The model under review builds one solid part; all positions refer to its coordinate system, in mm. A direction names the side the tool comes from. Give positions to 0.01 mm unless a question says otherwise; leave off trailing zeros. Loops run counter-clockwise (first coordinate to the right, second up) from the corner with the lowest first, then second, coordinate; pieces in that order, holes last. Notation, with made-up numbers: M 65.25,-28 L 109.25,-28 A19 cw 109.25,-9 Z; hole C -11,36 d11. An arc over 180 degrees is marked long. Return JSON: item names as keys, results as strings.
Autodesk Inventor part; units mm, degrees
ref_plane "YZ Plane" through (0, 0, 0) normal (1, 0, 0) x (0, 1, 0)
ref_plane "XZ Plane" through (0, 0, 0) normal (0, 1, 0) x (-1, 0, 0)
ref_plane "XY Plane" through (0, 0, 0) normal (0, 0, 1) x (1, 0, 0)
sketch "Sketch1" plane through (0, 0, 0) normal (0, 0, 1) x (1, 0, 0)
  line L0 (0, 0) -> (2, 0)
  line L1 (2, 0) -> (2, 10)
  line L2 (2, 10) -> (28, 10)
  line L3 (28, 10) -> (28, 0)
  line L4 (28, 0) -> (30, 0)
  line L5 (30, 0) -> (30, 12)
  line L6 (30, 12) -> (0, 12)
  line L7 (0, 12) -> (0, 0)
  line L8 (30, 15) -> (0, 15)
  dimension "d0" = 2
  dimension "d1" = 10
  dimension "d2" = 26
  dimension "d3" = 2
  dimension "d4" = 12
  dimension "d5" = 3
  dimension "d6" = 30
revolve "Revolution1" add sketch "Sketch1" angle 360 about axis through (30, 15, 0) along (-1, 0, 0)
sketch "Sketch2" plane through (0, 15, 0) normal (-1, 0, 0) x (0, 0, 1)
  circle A0 centre (7, 0) radius 2
  circle A1 centre (-7, 0) radius 2
  circle A2 centre (0, 7) radius 2
  circle A3 centre (0, -7) radius 2
  point P0 (0, -15)
  point P1 (0, 0)
  dimension "d8" = 4
  dimension "d10" = 4
  dimension "d13" = 4
  dimension "d14" = 4
  dimension "d17" = 7
  dimension "d18" = 7
  dimension "d19" = 7
  dimension "d20" = 7
sketch "Sketch3" plane through (0, 15, 0) normal (-1, 0, 0) x (0, 0, 1)
  point P0 (0, -15)
extrude "Extrusion1" cut sketch "Sketch2" against normal blind 2
sketch "Sketch4" plane through (30, 15, 0) normal (1, 0, 0) x (0, 0, -1)
  circle A0 centre (13, 0) radius 1
  circle A1 centre (-6, 0) radius 1
  point P0 (0, -15)
  point P1 (0, 0)
  dimension "d23" = 2
  dimension "d24" = 2
  dimension "d25" = 6
  dimension "d26" = 13
extrude "Extrusion2" cut sketch "Sketch4" against normal blind 2
properties part number "Spool1"
1) Insertion check: pin 1 (10 mm diameter, centred on y = 8, z = 4.5, fed in from -X); pin 2 (6 mm diameter, centred on x = 11.5, y = 6.5, fed in from -Z); pin 3 (2 mm diameter, centred on y = 8.5, z = -0.5, fed in from -X); pin 4 (5 mm diameter, centred on x = 24.5, z = -4, fed in from +Y). Each pin has a flat end and moves straight along its axis. Give the tip position at first contact, or say it passes through.
From the geometry:
{"pin 1": "x = 0", "pin 2": "through", "pin 3": "x = 28", "pin 4": "y = 19.77"}
2) Tool access review of faces 5 (the face through (29, 14, -13)), 6 (the face through (2, 19, 4)), 7 (the face through (1, 10, 0)), 8 (the face through (15, 18, 0)): name each direction out of +Z, -Z, +X, -X, +Y, -Y from which nothing blocks a thin tool from reaching the whole face with its end or side.
From the geometry:
{"face 5": "+X", "face 6": "none", "face 7": "-X", "face 8": "+X, -X"}
3) The part is to be moulded in two halves that separate along Y. For faces 1 (the face through (1, 17, 7)), 2 (the face through (0.986, 20.226, 0.923)), 3 (the face through (1, 27, 9)), 4 (the face through (30, 15, 4)), say which applies: released by +Y, released by -Y, zero draft, split by the parting line, or undercut.
From the geometry:
{"face 1": "undercut", "face 2": "undercut", "face 3": "split by the parting line", "face 4": "zero draft"}
4) Consider section C-C on y = 8. Write out the cut boundary in (x, z), then the cut area to 3 significant figures.
From the geometry:
{"outline": "M 0,-13.27 L 2,-13.27 L 2,-2 L 0,-2 Z; M 0,2 L 2,2 L 2,13.27 L 0,13.27 Z; M 28,-13.27 L 30,-13.27 L 30,13.27 L 28,13.27 Z", "area": "98.1 mm²"}
5) Consider section D-D on x = 22.25. Write out the cut boundary in (y, z).
From the geometry:
{"outline": "C 15,0 d10; hole C 15,0 d6"}
6) Consider section B-B on z = 8.25. Write out the cut boundary in (x, y), then the cut area to 3 significant figures.
From the geometry:
{"outline": "M 0,2.47 L 2,2.47 L 2,13.44 L 0,13.44 Z; M 0,16.56 L 2,16.56 L 2,27.53 L 0,27.53 Z; M 28,2.47 L 30,2.47 L 30,27.53 L 28,27.53 Z", "area": "94.0 mm²"}
7) Consider section A-A on z = 12. Write out the cut boundary in (x, y).
From the geometry:
{"outline": "M 0,6 L 2,6 L 2,24 L 0,24 Z; M 28,6 L 30,6 L 30,24 L 28,24 Z"}
8) Wall thickness on L1, parallel to Z at x = 0.65, y = 15; L2, parallel to X at y = 25.75, z = 3.5; L3, parallel to Z at x = 20.5, y = 15: over which ranges is each line inside the solid? List them lowest first. Write a range as from..to.
From the geometry:
{"L1": "-15..-9, -5..-3, 3..5, 9..15", "L2": "0..2, 28..30", "L3": "-5..-3, 3..5"}
